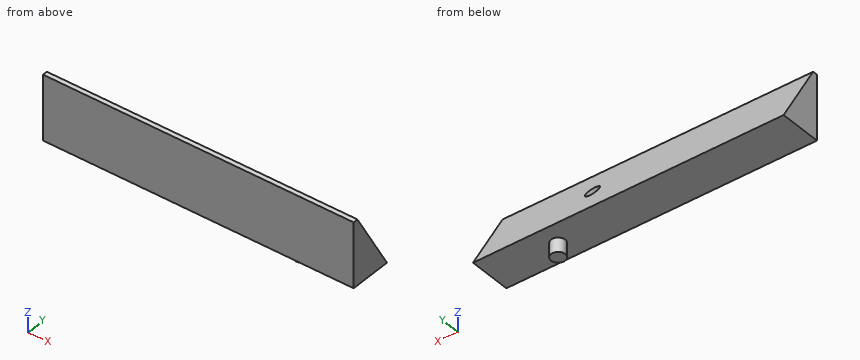
```python
from build123d import *

# Parameters (mm, degrees)
PAD_DEPTH    = 55
SKETCH001_R  = 2.5
PAD001_DEPTH = 5
SKETCH002_R  = 2.5
POCKET_DEPTH = 5


with BuildPart() as part:
    # Sketch → Pad (new body, symmetric)
    with BuildSketch(Plane.YZ):
        Polygon((0, 0), (-13.2790561914, 23), (-15, 23), (-15, 0), align=None)
    extrude(amount=PAD_DEPTH, both=True)

    # Sketch001 → Pad001 (join)
    with BuildSketch(Plane.XY):
        with Locations((30.7591449816, -7.5)):
            Circle(SKETCH001_R)
    extrude(amount=-PAD001_DEPTH)

    # Sketch002 (on Face1 of Pad001) → Pocket (cut)
    with BuildSketch(Plane(origin=(0, 0, 0), x_dir=(0, -0.5, 0.8660254038), z_dir=(0, 0.8660254038, 0.5))):
        with Locations((13.2790561914, 17.9531074876)):
            Circle(SKETCH002_R)
    extrude(amount=-POCKET_DEPTH, mode=Mode.SUBTRACT)


with BuildPart() as part_1:
    # Body placement: moved
    add(part.part.moved(Location((0, 15, 0))))


solid = part_1.part
```
Design review of the part built by this model. Coordinates are the model's own, in mm. Give positions to 0.01 mm unless a question says otherwise; leave off trailing zeros. Order: outer loops, then holes, each group sorted by start corner. A loop starts at its lowest first (then second) coordinate and runs counter-clockwise, first axis right, second up. Notation, with made-up numbers: M -18.5,-38 L 0.5,-38 A29 cw 0.5,-9 Z; hole C -11,-12 d1. An arc over 180 degrees is marked long. One line per question, with ' | ' between items. Start each with the question number.
Q1. For pin 1 Ø3 at (x, z) = (-32.5, -0.5) entering from -Y; pin 2 Ø8 at (x, y) = (-22, 9.5) entering from +Z; pin 3 Ø4.5 at (x, y) = (-5, 10.5) entering from -Z; pin 4 Ø5 at (x, y) = (-26.5, 6.5) entering from +Z, all flat-tipped, find the tip position at first contact; note any pin that passes through.
Q2. We need section B-B (z = 15.75). Write out the cut boundary in (x, y).
Q3. For L1, parallel to X at y = 7.5, z = 11; L2, parallel to Z at x = 38, y = 1.5; L3, parallel to X at y = 5.5, z = 10.5, list the stretches that pass through material, from the lowest coordinate up. Write a range as [from, to].
Q4. We need section A-A (x = -4). Write out the cut boundary in (y, z), plus the area to 3 significant figures.
Returned:
1) pin 1: y = 0 | pin 2: z = 16.45 | pin 3: z = 0 | pin 4: z = 19.05
2) outline: M -55,0 L 55,0 L 55,5.91 L -55,5.91 Z
3) L1: [-55, 15.45], [20.45, 55] | L2: [0, 23] | L3: [-55, 15.52], [20.39, 55]
4) outline: M 0,0 L 15,0 L 1.72,23 L 0,23 Z | area: 192 mm2
